Part model, mm, in its own coordinate system. A direction names the side the tool comes from. Coordinates: 2 decimals unless noted, no trailing zeros. Loops run counter-clockwise (first coordinate to the right, second up) from the corner with the lowest first, then second, coordinate; pieces in that order, holes last. Notation, with made-up numbers: M -19,48 L 31,48 A25 cw 31,83 Z; hole C -31,10 d8. An arc over 180 degrees is marked long. Answer as a JSON object with one key per item and string values. Group by question number.
1. Mould opens along Y. For faces 1 (the face through (-0.196, 1.487, 3.014)), 2 (the face through (0, 2, -6)), 3 (the face through (-1.5, 0.8, 4)) say: released by +Y, released by -Y, zero draft, split by the parting line, or undercut.
2. Drop flat-ended pins along their axis: pin 1 Ø2 at (y, z) = (1.5, -10) entering from +X; pin 2 Ø1 at (y, z) = (-1.5, -6.5) entering from -X. Give the stop position or say it passes through.
3. 3-axis set-ups, long thin cutter, end or side, ignore diameter. For faces 4 (the face through (1, -2, 0)), 5 (the face through (0, 0, -12)), 6 (the face through (-1.386, 0.574, 3.014)): which of +Z, -Z, +X, -X, +Y, -Y reach the whole face in a straight line?
4. Saw through at C-C on z = -9.25. Write the cut outline in (x, y).
5. Saw through at B-B on x = 0. Write the cut outline in (y, z).
6. Drill centre lines: L1, parallel to Z at x = 2, y = -2.5; L2, parallel to X at y = 0, z = -6. Where is each one in solid material? Low to high.
7. Saw through at A-A on y = 0. Write the cut outline in (x, z), then the cut area to 3 significant figures.
from build123d import *

# Parameters (mm, degrees)
F0_R     = 3.5
F1_DEPTH = 4
F3_DEPTH = 2
F4_R     = 2
F5_DEPTH = 12
F6_SIZE  = 0.5
F7_SIZE  = 0.25


with BuildPart() as f1:
    # F0 (on Top) → F1 (new body)
    with BuildSketch(Plane.XY):
        Circle(F0_R)
    extrude(amount=F1_DEPTH)

    # F2 (on face) → F3 (cut)
    with BuildSketch(Plane.XY.offset(4)):
        Polygon((1.0656559782, -1.3654220359), (1.7153181591, 0.2401741309), (0.6496621809, 1.6055961668), (-1.0656559782, 1.3654220359), (-1.7153181591, -0.2401741309), (-0.6496621809, -1.6055961668), align=None)
    extrude(amount=-F3_DEPTH, mode=Mode.SUBTRACT)

    # F4 (on face) → F5 (join)
    with BuildSketch(Plane(origin=(0, 0, 0), x_dir=(1, 0, 0), z_dir=(0, 0, -1))):
        Circle(F4_R)
    extrude(amount=F5_DEPTH)

    # F6
    f6_edges = [f1.edges().sort_by_distance(p)[0] for p in [
        (-2, 0, -12),
    ]]
    chamfer(f6_edges, length=F6_SIZE)

    # F7
    f7_edges = [f1.edges().sort_by_distance(p)[0] for p in [
        (-3.5, 0, 0),
        (-3.5, 0, 4),
    ]]
    chamfer(f7_edges, length=F7_SIZE)


solid = f1.part
Outcome:
{
 "1": {"face 1": "undercut", "face 2": "split by the parting line", "face 3": "zero draft"},
 "2": {"pin 1": "stops at x = 1.94", "pin 2": "stops at x = -1.73"},
 "3": {"face 4": "-Z", "face 5": "-Z, +X, -X, +Y, -Y", "face 6": "+Z"},
 "4": {"outline": "C 0,0 d4"},
 "5": {"outline": "M -3.5,0.25 L -3.25,0 L -2,0 L -2,-11.5 L -1.5,-12 L 1.5,-12 L 2,-11.5 L 2,0 L 3.25,0 L 3.5,0.25 L 3.5,3.75 L 3.25,4 L 1.51,4 L 1.51,2 L -1.51,2 L -1.51,4 L -3.25,4 L -3.5,3.75 Z"},
 "6": {"L1": "z = 0 to 4", "L2": "x = -2 to 2"},
 "7": {"outline": "M -3.5,0.25 L -3.25,0 L -2,0 L -2,-11.5 L -1.5,-12 L 1.5,-12 L 2,-11.5 L 2,0 L 3.25,0 L 3.5,0.25 L 3.5,3.75 L 3.25,4 L 1.62,4 L 1.62,2 L -1.62,2 L -1.62,4 L -3.25,4 L -3.5,3.75 Z", "area": "69.2 mm²"}
}
